Source: CAD feature listing. Evaluate the final solid. Frame: model axes, mm. Face numbers are marked on the shaded views. A direction names the side the tool comes from. Give positions to 0.01 mm unless a question says otherwise; leave off trailing zeros. Loops run counter-clockwise (first coordinate to the right, second up) from the corner with the lowest first, then second, coordinate; pieces in that order, holes last.
```python
from build123d import *

# Parameters (mm, degrees)
SKETCH2_R               = 5
BOSS_EXTRUDE1_DEPTH     = 7
SKETCH3_R               = 3
BOSS_EXTRUDE2_DEPTH     = 30.5
SKETCH4_R               = 1.5
CUT_EXTRUDE1_DEPTH      = 3
CUT_EXTRUDE2_DEPTH      = 4
CUT_EXTRUDE2_DEPTH_BACK = 4
SKETCH5_R               = 1.5
CHAMFER1_SIZE           = 0.5
FILLET1_R               = 0.5
CHAMFER2_SIZE           = 0.5
CHAMFER3_SIZE           = 0.5
FILLET4_R               = 1


with BuildPart() as part:
    # Sketch1 → Revolve1 (revolve)
    with BuildSketch(Plane.XY, mode=Mode.PRIVATE) as revolve1_sk:
        Polygon((0, 67), (18.5, 67), (18.5, 40), (13.75, 40), (13.75, 2), (4, 2), (4, 0), (0, 0), align=None)
    revolve(revolve1_sk.sketch.rotate(Axis((0, 116.312873798, 0), (0, -1, 0)), 90), axis=Axis((0, 116.312873798, 0), (0, -1, 0)))

    # Sketch2 → Boss-Extrude1 (add)
    with BuildSketch(Plane(origin=(0, 67, 0), x_dir=(1, 0, 0), z_dir=(0, 1, 0))):
        with Locations(Location((-8.140754401, 0, 0), (0, 0, 90))):
            Circle(SKETCH2_R)
    extrude(amount=BOSS_EXTRUDE1_DEPTH)

    # Sketch3 → Boss-Extrude2 (add)
    with BuildSketch(Plane(origin=(0, 74, 0), x_dir=(1, 0, 0), z_dir=(0, 1, 0))):
        with Locations(Location((-8.140754401, 0, 0), (0, 0, 90))):
            Circle(SKETCH3_R)
    extrude(amount=BOSS_EXTRUDE2_DEPTH)

    # Sketch4 → Cut-Extrude1 (cut)
    with BuildSketch(Plane(origin=(0, 67, 0), x_dir=(1, 0, 0), z_dir=(0, 1, 0))):
        with Locations(Location((0, 15.25, 0), (0, 0, 270))):
            Circle(SKETCH4_R)
        with Locations(Location((13.206887408, 7.625, 0), (0, 0, 270))):
            Circle(SKETCH4_R)
        with Locations(Location((13.206887408, -7.625, 0), (0, 0, 270))):
            Circle(SKETCH4_R)
        with Locations(Location((0, -15.25, 0), (0, 0, 270))):
            Circle(SKETCH4_R)
        with Locations(Location((-13.206887408, -7.625, 0), (0, 0, 270))):
            Circle(SKETCH4_R)
        with Locations(Location((-13.206887408, 7.625, 0), (0, 0, 270))):
            Circle(SKETCH4_R)
    extrude(amount=-CUT_EXTRUDE1_DEPTH, mode=Mode.SUBTRACT)

    # Sketch5 → Cut-Extrude2 (cut, two sides: drawn at the far end of the back side and taken through both)
    with BuildSketch(Plane.XY.offset(-CUT_EXTRUDE2_DEPTH_BACK)):
        with Locations(Location((-8.140754401, 98.6, 0), (0, 0, 89.99999999))):
            Circle(SKETCH5_R)
    extrude(amount=CUT_EXTRUDE2_DEPTH + CUT_EXTRUDE2_DEPTH_BACK, mode=Mode.SUBTRACT)

    # Chamfer1
    chamfer1_edges = [part.edges().sort_by_distance(p)[0] for p in [
        (-8.140754401, 67, 5),
        (-8.140754401, 74, 5),
    ]]
    chamfer(chamfer1_edges, length=CHAMFER1_SIZE)

    # Fillet1
    fillet1_edges = [part.edges().sort_by_distance(p)[0] for p in [
        (0, 0, -4),
    ]]
    fillet(fillet1_edges, radius=FILLET1_R)

    # Chamfer2
    chamfer2_edges = [part.edges().sort_by_distance(p)[0] for p in [
        (0, 2, -4),
    ]]
    chamfer(chamfer2_edges, length=CHAMFER2_SIZE)

    # Chamfer3
    chamfer3_edges = [part.edges().sort_by_distance(p)[0] for p in [
        (-8.140754401, 104.5, 3),
    ]]
    chamfer(chamfer3_edges, length=CHAMFER3_SIZE)

    # Fillet4
    fillet4_edges = [part.edges().sort_by_distance(p)[0] for p in [
        (0, 67, -18.5),
    ]]
    fillet(fillet4_edges, radius=FILLET4_R)

    # Sketch6 → Cut-Revolve1 (revolve, cut)
    with BuildSketch(Plane.XY, mode=Mode.PRIVATE) as cut_revolve1_sk:
        with BuildLine():
            Line((13.769543402, 40), (12.269543402, 40))
            ThreePointArc((12.269543402, 40), (13.330203573, 39.560660172), (13.769543402, 38.5))
            Line((13.769543402, 38.5), (13.769543402, 40))
        make_face()
    revolve(cut_revolve1_sk.sketch.rotate(Axis((0, 116.312873798, 0), (0, -1, 0)), 90), axis=Axis((0, 116.312873798, 0), (0, -1, 0)), mode=Mode.SUBTRACT)


solid = part.part
```
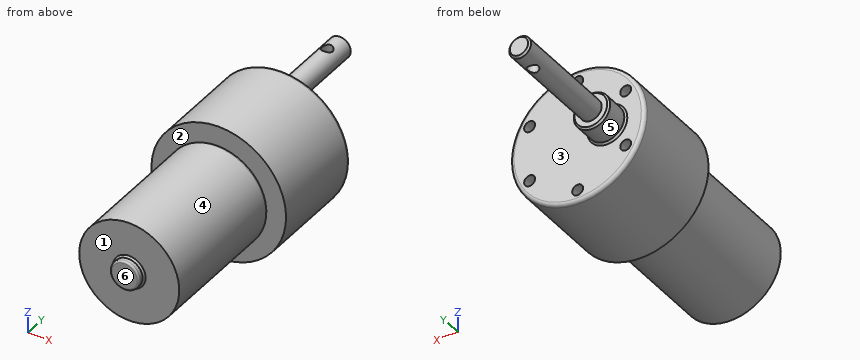
(1) Section A-A, the plane y = 98.6. Return the cut outline in (x, z).
A:
outline: (-9.64, -2.6) - (-9.64, 2.6) arc R3 ccw to start; (-6.64, -2.6) arc R3 ccw to (-6.64, 2.6) - close
(2) Ray query, line 1 along Y through (x, z) = (-4.5, -10); line 2 along X through (y, z) = (65.3, 15.25); line 3 along Y through (x, z) = (-14.5, 8.5). Return the intervals inside material, ascending.
A:
line 1: y = 2 to 67
line 2: x = -10.47 to -1.5, 1.5 to 10.47
line 3: y = 40 to 67
(3) Section D-D, the plane y = 11. Return the cut outline in (x, z).
A:
outline: circle Ø27.5 at (0, 0)
(4) Reachability of the marked faces 5 and 6 from +Z, -Z, +X, -X, +Y, -Y: full face, straight path, thin tool, end or side. Return the list, or none.
A:
face 5: +Y
face 6: +Z, -Z, +X, -X, -Y
(5) First-contact query: pin 1 (5 mm diameter, centred on x = -12, z = 6.5, fed in from -Y); pin 2 (4 mm diameter, centred on x = 13.21, z = -7.62, fed in from +Y); pin 3 (1.5 mm diameter, centred on y = 24.5, z = 0.5, fed in from +X). Flat tips, straight axial feed; report the tip coordinate or a pass-through.
A:
pin 1: stops at y = 2
pin 2: stops at y = 67
pin 3: stops at x = 13.75
(6) Section B-B, the plane x = 0. Return the cut outline in (y, z).
A:
outline: (0, -3.5) arc R0.5 ccw to (0.5, -4) - (1.5, -4) - (2, -4.5) - (2, -13.75) - (38.74, -13.75) arc R1.5 ccw to (40, -12.27) - (40, -18.5) - (66, -18.5) arc R1 ccw to (67, -17.5) - (67, -16.75) - (64, -16.75) - (64, -13.75) - (67, -13.75) - (67, 13.75) - (64, 13.75) - (64, 16.75) - (67, 16.75) - (67, 17.5) arc R1 ccw to (66, 18.5) - (40, 18.5) - (40, 12.27) arc R1.5 ccw to (38.74, 13.75) - (2, 13.75) - (2, 4.5) - (1.5, 4) - (0.5, 4) arc R0.5 ccw to (0, 3.5) - close
(7) Mould query, pull axis Y, two halves, no side actions, for the marked faces 1, 2, 3 and 4. Classes: pulls with the +Y half, pulls with the -Y half, needs draft (parallel to the pull), parting line crosses it, or undercut.
A:
face 1: pulls with the -Y half
face 2: undercut
face 3: pulls with the +Y half
face 4: needs draft
(8) Section C-C, the plane y = 52. Return the cut outline in (x, z), then the cut area to 3 significant figures.
A:
outline: circle Ø37 at (0, 0)
area: 1,080 mm2
